from build123d import *

# Parameters (mm, degrees)
EXTRUDE_420_DEPTH          = 22
SKETCH_473_W               = 6
SKETCH_473_H               = 8
EXTRUDE_540_DEPTH          = 5.9
SKETCH_591_W               = 5
SKETCH_591_H               = 5
EXTRUDE_711_DEPTH          = 5.9
CUT_EXTRUDE_4_DEPTH        = 54.062321849
CUT_EXTRUDE_4_DEPTH_BACK   = 54.062321849
SKETCH_4_R                 = 2.25
CUT_EXTRUDE_4_2_DEPTH      = 49.538644398
CUT_EXTRUDE_4_2_DEPTH_BACK = 49.538644398
SKETCH_4_2_R               = 2.25
CUT_EXTRUDE_4_3_DEPTH      = 3.4
CUT_EXTRUDE_4_4_DEPTH      = 54.062321849
CUT_EXTRUDE_4_4_DEPTH_BACK = 54.062321849
SKETCH_4_4_W               = 3.4
SKETCH_4_4_H               = 7.35


with BuildPart() as part:
    # Sketch 413 → Extrude 420 (new body)
    with BuildSketch(Plane.XY):
        Polygon((0, 0), (18, 0), (18, 11.5), (36, 11.5), (36, 24), (0, 24), align=None)
    extrude(amount=EXTRUDE_420_DEPTH)

    # Sketch 473 → Extrude 540 (add)
    with BuildSketch(Plane(origin=(0, 0, 0), x_dir=(1, 0, 0), z_dir=(0, 1, 0))):
        with Locations((13, -11)):
            Rectangle(SKETCH_473_W, SKETCH_473_H)
    extrude(amount=-EXTRUDE_540_DEPTH)

    # Sketch 591 → Extrude 711 (add)
    with BuildSketch(Plane(origin=(36, 0, 0), x_dir=(0, 0, -1), z_dir=(1, 0, 0))):
        with Locations((-4.5, 18.5)):
            Rectangle(SKETCH_591_W, SKETCH_591_H)
    extrude(amount=EXTRUDE_711_DEPTH)

    # Sketch 4 → Cut-Extrude 4 (cut, two sides: drawn at the far end of the back side and taken through both)
    with BuildSketch(Plane(origin=(0, 0, 0), x_dir=(1, 0, 0), z_dir=(0, 1, 0)).offset(-CUT_EXTRUDE_4_DEPTH_BACK)):
        with Locations(Location((5, -11, 0), (0, 0, 270))):
            Circle(SKETCH_4_R)
    extrude(amount=CUT_EXTRUDE_4_DEPTH + CUT_EXTRUDE_4_DEPTH_BACK, mode=Mode.SUBTRACT)

    # Sketch 4 2 → Cut-Extrude 4 2 (cut, two sides: drawn at the far end of the back side and taken through both)
    with BuildSketch(Plane(origin=(36, 0, 0), x_dir=(0, 0, -1), z_dir=(1, 0, 0)).offset(-CUT_EXTRUDE_4_2_DEPTH_BACK)):
        with Locations(Location((-11, 17.5, 0), (0, 0, 180))):
            Circle(SKETCH_4_2_R)
    extrude(amount=CUT_EXTRUDE_4_2_DEPTH + CUT_EXTRUDE_4_2_DEPTH_BACK, mode=Mode.SUBTRACT)

    # Sketch 4 3 → Cut-Extrude 4 3 (cut)
    with BuildSketch(Plane(origin=(0, 24, 0), x_dir=(1, 0, 0), z_dir=(0, 1, 0))):
        Polygon((9.243524479, -11), (7.121762239, -14.675), (2.878237761, -14.675), (0.756475521, -11), (2.878237761, -7.325), (7.121762239, -7.325), align=None)
    extrude(amount=-CUT_EXTRUDE_4_3_DEPTH, mode=Mode.SUBTRACT)

    # Sketch 4 4 → Cut-Extrude 4 4 (cut, two sides: drawn at the far end of the back side and taken through both)
    with BuildSketch(Plane.XY.offset(-CUT_EXTRUDE_4_4_DEPTH_BACK)):
        with Locations((25.7, 17.5)):
            Rectangle(SKETCH_4_4_W, SKETCH_4_4_H)
    extrude(amount=CUT_EXTRUDE_4_4_DEPTH + CUT_EXTRUDE_4_4_DEPTH_BACK, mode=Mode.SUBTRACT)


solid = part.part
Build history of the part. All positions in model axes, mm. A direction names the side the tool comes from. Round coordinates to 2 decimals unless told otherwise and drop trailing zeros. Write each loop counter-clockwise with the first axis right and the second up, starting at its lowest first coordinate (ties: lowest second). Pieces come first, ordered by that corner, then holes. Notation, with made-up numbers: M 29,42.5 L 60,42.5 A13 ccw 60,64.5 Z; hole C 14.25,1.25 d11. An arc over 180 degrees is marked long. Answer as a JSON object with one key per item and string values. Group by question number.
(1) Flat gauge pins, fed straight in: pin 1 (4 mm diameter, centred on x = 40.5, y = 18.5, fed in from +Z); pin 2 (5.5 mm diameter, centred on x = 39.5, z = 3.5, fed in from -Y); pin 3 (12.5 mm diameter, centred on y = 5, z = 8, fed in from +X); pin 4 (2.5 mm diameter, centred on x = 5, z = 11, fed in from +Y). Where does each tip first touch, or does it go through?
(2) Drill centre lines: L1, parallel to X at y = 4.5, z = 11; L2, parallel to Z at x = 5, y = 19.75; L3, parallel to X at y = -0.75, z = 10.75. Where is each one in solid material? Low to high.
(3) Cut at A-A (z = 18.75). Give the cut face in (x, y) (3 decimals).
(4) Cut at B-B (x = 4). Give the cut face in (y, z) (3 decimals).
(5) Which spindle directions (+Z, -Z, +X, -X, +Y, -Y) get a long thin tool onto all of the face, cutting with end or side? Do faces 1 (the flat face through (13, -3, 15)), 2 (the flat face through (39, 18, 7)), 3 (the flat face through (18, 6, 11)), 4 (the flat face through (1.8, 22.32, 9.19)). Say none if no direction does.
(6) Cut at C-C (y = 7.25). Give the cut face in (x, z).
(7) Mould opens along Y. For faces 5 (the flat face through (26, 21.175, 11)), 6 (the flat face through (8.2, 22.32, 12.81)), 7 (the flat face through (39, 16, 5)) say: pulls with the +Y half, pulls with the -Y half, needs draft (parallel to the pull), parting line crosses it, or undercut.
(8) Cut at D-D (x = 35.5). Give the cut face in (y, z).
Responses:
{
 "1": {"pin 1": "stops at z = 7", "pin 2": "stops at y = 16", "pin 3": "stops at x = 18", "pin 4": "passes through"},
 "2": {"L1": "x = 0 to 2.75, 7.25 to 18", "L2": "z = 0 to 8.75, 13.25 to 22", "L3": "x = 10 to 16"},
 "3": {"outline": "M 0,0 L 18,0 L 18,11.5 L 36,11.5 L 36,24 L 0,24 Z; hole M 24,13.825 L 27.4,13.825 L 27.4,21.175 L 24,21.175 Z"},
 "4": {"outline": "M 0,0 L 24,0 L 24,7.325 L 20.6,7.325 L 20.6,8.984 L 18.5,8.984 A2.25 cw 16.5,8.984 L 0,8.984 Z; M 0,13.016 L 16.5,13.016 A2.25 cw 18.5,13.016 L 20.6,13.016 L 20.6,14.675 L 24,14.675 L 24,22 L 0,22 Z"},
 "5": {"face 1": "+Z, +X, -X, -Y", "face 2": "+Z, +X, +Y, -Y", "face 3": "+Z, -Z, +X, -Y", "face 4": "+Y"},
 "6": {"outline": "M 0,0 L 18,0 L 18,22 L 0,22 Z; hole C 5,11 d4.5"},
 "7": {"face 5": "undercut", "face 6": "needs draft", "face 7": "pulls with the -Y half"},
 "8": {"outline": "M 11.5,0 L 24,0 L 24,22 L 11.5,22 Z; hole C 17.5,11 d4.5"}
}
